Autodesk Inventor part; units mm, degrees
ref_plane "YZ Plane" through (0, 0, 0) normal (1, 0, 0) x (0, 1, 0)
ref_plane "XZ Plane" through (0, 0, 0) normal (0, 1, 0) x (-1, 0, 0)
ref_plane "XY Plane" through (0, 0, 0) normal (0, 0, 1) x (1, 0, 0)
sketch "Sketch1" plane through (0, 0, 0) normal (0, 0, 1) x (1, 0, 0)
  line L0 (-85, 0) -> (85, 0)
  line L1 (85, 0) -> (85, 100)
  line L2 (85, 100) -> (-85, 100)
  line L3 (-85, 100) -> (-85, 0)
  point P0 (0, 0)
  point P1 (0, 0)
  dimension "d0" = 170
  dimension "d1" = 100
extrude "Extrusion1" add sketch "Sketch1" along normal blind 4
sketch "Sketch2" plane through (-85, 0, 0) normal (0, -1, 0) x (1, 0, 0)
  line L0 (170, 4) -> (0, 4)
  line L1 (170, 0) -> (0, 0)
  line L2 (60, 4) -> (110, 4)
  line L3 (110, 4) -> (110, 0)
  line L4 (110, 0) -> (60, 0)
  line L5 (60, 0) -> (60, 4)
  point P0 (85, 0)
  point P1 (85, 0)
  dimension "d4" = 25
  dimension "d5" = 50
extrude "Extrusion2" add sketch "Sketch2" along normal blind 4
sketch "Sketch4" plane through (0, 0, 4) normal (0, 0, 1) x (1, 0, 0)
  line L0 (85, 0) -> (85, 100)
  line L1 (85, 35) -> (81, 35)
  line L2 (81, 35) -> (81, 65)
  line L3 (81, 65) -> (85, 65)
  line L4 (85, 65) -> (85, 35)
  line L5 (85, 100) -> (-85, 100)
  line L6 (25, 0) -> (85, 0)
  point P0 (0, 0)
  dimension "d12" = 4
  dimension "d13" = 35
  dimension "d14" = 35
extrude "Extrusion4" cut sketch "Sketch4" against normal blind 10
mirror "Mirror2" about plane through (0, 0, 0) normal (1, 0, 0) of "Extrusion4"
sketch "Sketch5" plane through (-85, 100, 0) normal (0, 1, 0) x (1, 0, 0)
  line L0 (170, -4) -> (0, -4)
  line L1 (45, 0) -> (125, 0)
  line L2 (125, 0) -> (125, -4)
  line L3 (125, -4) -> (45, -4)
  line L4 (45, -4) -> (45, 0)
  line L5 (170, 0) -> (0, 0)
  point P0 (85, 0)
  point P1 (85, 0)
  point P2 (45, -4)
  dimension "d17" = 80
  dimension "d18" = 40
extrude "Extrusion5" cut sketch "Sketch5" against normal blind 4
sketch "Sketch6" plane through (0, 0, 4) normal (0, 0, 1) x (1, 0, 0)
  line L0 (-30, 54) -> (30, 54)
  line L1 (30, 54) -> (30, 50)
  line L2 (30, 50) -> (-30, 50)
  line L3 (-30, 50) -> (-30, 54)
  point P0 (0, 0)
  point P1 (0, 54)
  dimension "d21" = 60
  dimension "d22" = 4
  dimension "d23" = 50
extrude "Extrusion6" cut sketch "Sketch6" against normal blind 10
properties part number "Tapa Tracera"
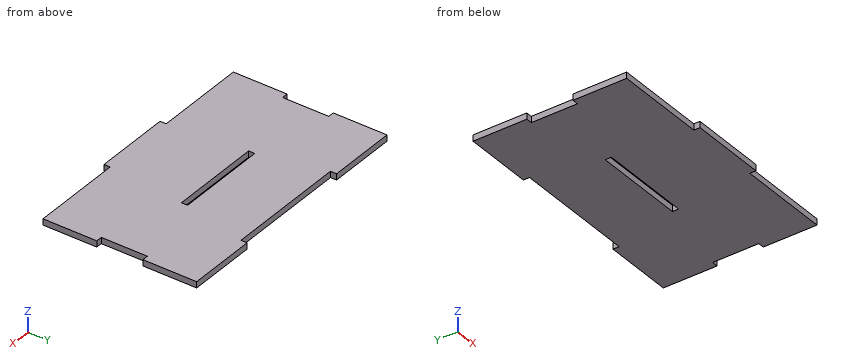
For this review, take the finished solid that the model builds, in its own axes (mm). Give positions to 0.01 mm unless a question says otherwise; leave off trailing zeros. Loops run counter-clockwise (first coordinate to the right, second up) from the corner with the lowest first, then second, coordinate; pieces in that order, holes last. Notation, with made-up numbers: M -14,67 L 28,67 A26 cw 28,92 Z; hole C -2,68 d10. An arc over 180 degrees is marked long. Put each result on its own line as item: value. Start each with the question number.
(1) Wall thickness on L1, parallel to Y at x = 2, z = 1.9; L2, parallel to Y at x = -74, z = 1.05; L3, parallel to Y at x = 34.5, z = 0.5: over which ranges is each line inside the solid? List them lowest first.
(2) Add section D-D, the plane x = -37. Write out the cut boundary in (y, z), then the cut area to 3 significant figures.
(3) Add section A-A, the plane x = 11. Write out the cut boundary in (y, z).
(4) Add section B-B, the plane z = 2.15. Write out the cut boundary in (x, y).
(5) For pin 1 (1 mm diameter, centred on x = 45.5, z = 1.5, fed in from -Y); pin 2 (2 mm diameter, centred on x = 3, z = 1, fed in from +Y); pin 3 (1.2 mm diameter, centred on y = 56.5, z = 3, fed in from -X), all flat-tipped, find the tip position at first contact; note any pin that passes through.
(6) Add section C-C, the plane y = 40. Write out the cut boundary in (x, z).
Result:
1. L1: y = -4 to 50, 54 to 96
1. L2: y = 0 to 100
1. L3: y = 0 to 96
2. outline: M 0,0 L 96,0 L 96,4 L 0,4 Z
2. area: 384 mm^2
3. outline: M -4,0 L 50,0 L 50,4 L -4,4 Z; M 54,0 L 96,0 L 96,4 L 54,4 Z
4. outline: M -85,0 L -25,0 L -25,-4 L 25,-4 L 25,0 L 85,0 L 85,35 L 81,35 L 81,65 L 85,65 L 85,100 L 40,100 L 40,96 L -40,96 L -40,100 L -85,100 L -85,65 L -81,65 L -81,35 L -85,35 Z; hole M -30,50 L 30,50 L 30,54 L -30,54 Z
5. pin 1: stops at y = 0
5. pin 2: stops at y = 96
5. pin 3: stops at x = -81
6. outline: M -81,0 L 81,0 L 81,4 L -81,4 Z
